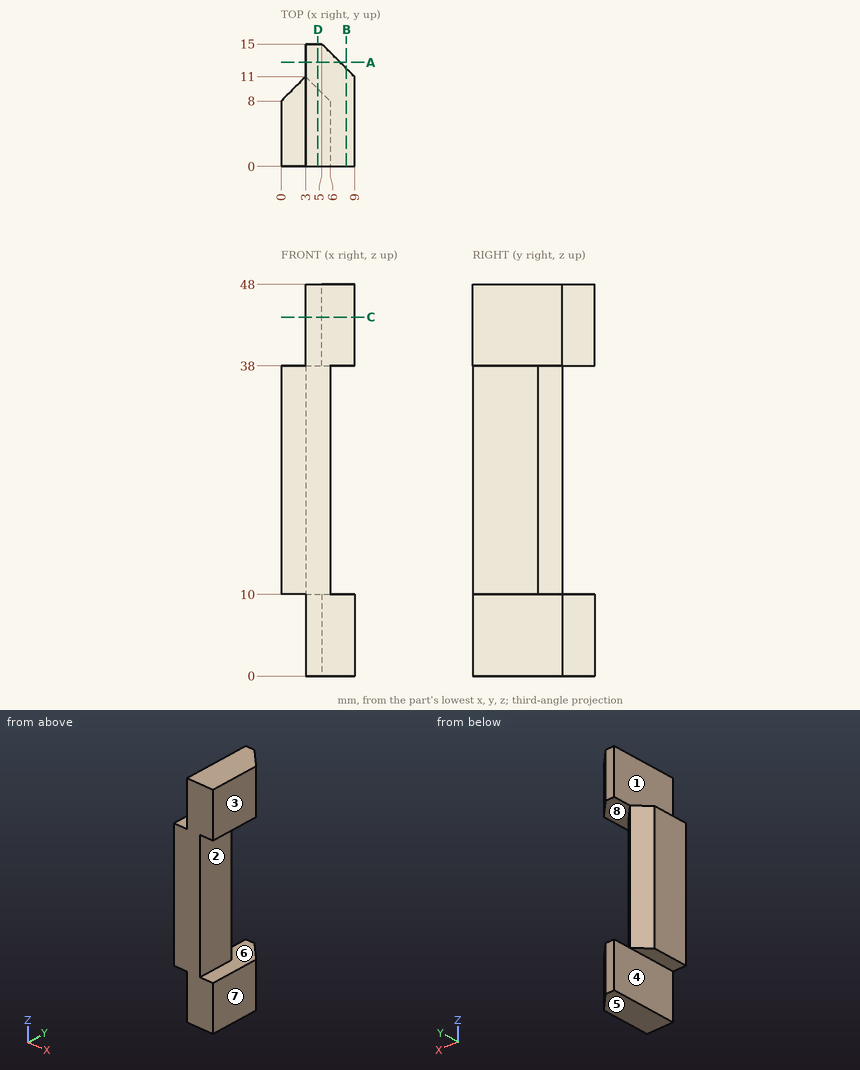
Design review of the part shown in the three views and the two pictorial views. Dimensions are in mm from the part's minimum x, y and z. A direction names the side the tool comes from. Round coordinates to 2 decimals unless told otherwise and drop trailing zeros. Write each loop counter-clockwise with the first axis right and the second up, starting at its lowest first coordinate (ties: lowest second). Pieces come first, ordered by that corner, then holes.
Item 1: Clearance check with flat-ended pins moving along their axes: pin 1 Ø0.9 at (x, y) = (2, 3) entering from -Z; pin 2 Ø9 at (y, z) = (5.5, 23.5) entering from +X; pin 3 Ø3 at (y, z) = (11, 42) entering from -X. State where each tip first meets the part, or that it passes through.
Item 2: We need section D-D on x = 4.5. Write out the cut boundary in (y, z).
Item 3: For the marked faces 1, 2, 3 and 4, list the 3-axis set-ups (+Z, -Z, +X, -X, +Y, -Y) from which the entire face can be reached by the end or side of a thin tool; tool diameter is ignored.
Item 4: We need section B-B on x = 8. Write out the cut boundary in (y, z), and give its area (3 significant figures).
Item 5: We need section C-C on z = 44. Write out the cut boundary in (x, y).
Item 6: We need section A-A on y = 12.75. Write out the cut boundary in (x, z), and give its area (3 significant figures).
Item 7: The part is to be moulded in two halves that separate along Z. For the marked faces 5, 6, 7 and 8, say which applies: +Z half, -Z half, draft (parallel to the pull), parting line (faces both ways), or undercut.
Item 8: For probe 1 along Z at (x, y) = (3.25, 13.75); probe 2 along Z at (x, y) = (0.5, 4.25); probe 3 along X at (y, z) = (4, 13.5), list the stretches that pass through material, from the lowest coordinate up.
Returned:
1. pin 1: stops at z = 10
1. pin 2: stops at x = 6
1. pin 3: stops at x = 3
2. outline: (0, 0) - (15, 0) - (15, 10) - (9.5, 10) - (9.5, 38) - (15, 38) - (15, 48) - (0, 48) - close
3. face 1: +Z, -X, +Y, -Y
3. face 2: +X, +Y, -Y
3. face 3: +Z, -Z, +X, +Y, -Y
3. face 4: -Z, -X, +Y, -Y
4. outline: (0, 0) - (12, 0) - (12, 10) - (0, 10) - close; (0, 38) - (12, 38) - (12, 48) - (0, 48) - close
4. area: 240 mm2
5. outline: (3, 0) - (9, 0) - (9, 11) - (5, 15) - (3, 15) - close
6. outline: (3, 0) - (7.25, 0) - (7.25, 10) - (3, 10) - close; (3, 38) - (7.25, 38) - (7.25, 48) - (3, 48) - close
6. area: 85.0 mm2
7. face 5: -Z half
7. face 6: undercut
7. face 7: draft
7. face 8: undercut
8. probe 1: z = 0 to 10, 38 to 48
8. probe 2: z = 10 to 38
8. probe 3: x = 0 to 6
